from build123d import *


with BuildPart() as part:
    # Sketch2 → Revolve1 (revolve)
    with BuildSketch(Plane.XY):
        with BuildLine():
            Line((-13.5, 40), (-13.5, 15))
            ThreePointArc((-13.5, 15), (-9.545941546, 5.454058454), (0, 1.5))
            Line((0, 1.5), (0, 0))
            ThreePointArc((0, 0), (-10.606601718, 4.393398282), (-15, 15))
            Line((-15, 15), (-15, 37.935568233))
            Line((-15, 37.935568233), (-17.985762804, 37.935568233))
            Line((-17.985762804, 37.935568233), (-17.985762804, 40))
            Line((-17.985762804, 40), (-15, 40))
            Line((-15, 40), (-13.5, 40))
        make_face()
    revolve(axis=Axis((0, 107.077522155, 0), (0, -1, 0)))


solid = part.part
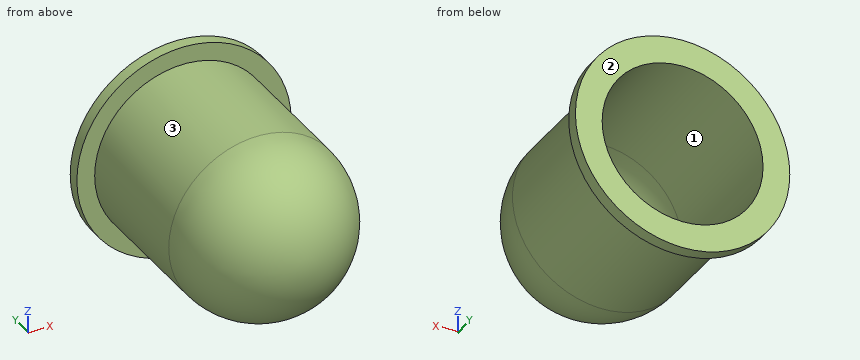
Geometry check sheet. Reference: the model listing, model coordinates, mm. Face numbers are marked on the shaded views. Round coordinates to 2 decimals unless told otherwise and drop trailing zeros. Order: outer loops, then holes, each group sorted by start corner. A loop starts at its lowest first (then second) coordinate and runs counter-clockwise, first axis right, second up. Notation, with made-up numbers: M 63,33.5 L 121,33.5 A29 cw 121,64.5 Z; hole C 49.25,30 d8. An arc over 180 degrees is marked long. Write each question's results on one line, items separated by ' | '. Start each with the question number.
1. Material ranges on L1, parallel to Z at x = 0, y = 31; L2, parallel to Y at x = 12, z = -10, recorded low to high. Write a range as from..to.
2. Go/stop test with flat-tipped pins: P1, Ø1, axis at x = -2, z = -4, coming from the +Y side; P2, Ø11, axis at x = 0.5, z = -7.5, coming from the -Y side; P3, Ø6, axis at y = 19, z = -12.5, coming from the +X side. Record where each tip stops, or that it passes through.
3. Cross-section at C-C on y = 6. Record the boundary of the cut face in (x, z).
4. Draft check along Z on the marked faces 1, 2 and 3. Enter one of: pulls with the +Z half, pulls with the -Z half, needs draft (parallel to the pull), parting line crosses it, or undercut.
5. Cross-section at D-D on z = -6.5. Record the boundary of the cut face in (x, y).
6. Cross-section at A-A on z = 0. Record the boundary of the cut face in (x, y), plus the area to 3 significant figures.
7. Cross-section at B-B on x = 0. Record the boundary of the cut face in (y, z), plus the area to 3 significant figures.
Resolved:
1) L1: -15..-13.5, 13.5..15 | L2: 37.94..40
2) P1: y = 2.45 | P2: y = 0.14 | P3: x = 11.61
3) outline: C 0,0 d24; hole C 0,0 d20.12
4) face 1: undercut | face 2: needs draft | face 3: parting line crosses it
5) outline: M -16.77,37.94 L -13.52,37.94 L -13.52,15 A13.52 ccw 13.52,15 L 13.52,37.94 L 16.77,37.94 L 16.77,40 L 11.83,40 L 11.83,15 A11.83 cw -11.83,15 L -11.83,40 L -16.77,40 Z
6) outline: M -17.99,37.94 L -15,37.94 L -15,15 A15 ccw 15,15 L 15,37.94 L 17.99,37.94 L 17.99,40 L 13.5,40 L 13.5,15 A13.5 cw -13.5,15 L -13.5,40 L -17.99,40 Z | area: 154 mm2
7) outline: M 15,-15 L 37.94,-15 L 37.94,-17.99 L 40,-17.99 L 40,-13.5 L 15,-13.5 A13.5 cw 15,13.5 L 40,13.5 L 40,17.99 L 37.94,17.99 L 37.94,15 L 15,15 A15 ccw Z | area: 154 mm2
